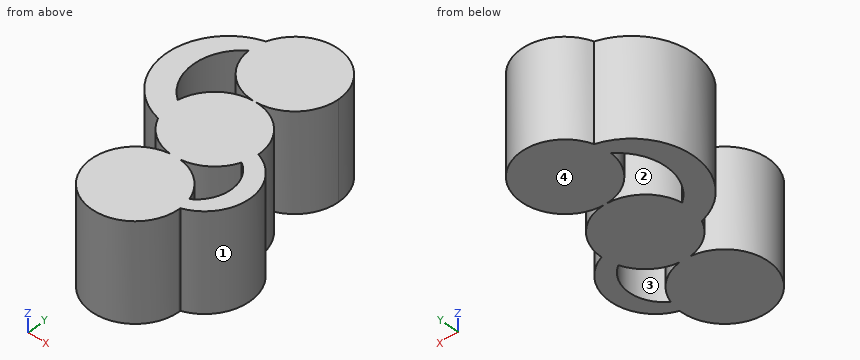
from build123d import *

# Parameters (mm, degrees)
F1_DEPTH = 25


with BuildPart() as f1:
    # F0 (on Top) → F1 (new body)
    with BuildSketch(Plane.XY):
        with BuildLine():
            ThreePointArc((-0.3111750606, 11.1956764013), (-7.4017548814, 8.4055948436), (-11.0663750249, 1.7249184932))
            ThreePointArc((-11.0663750249, 1.7249184932), (-11.0810170285, -1.6282080989), (-10.1024246207, -4.8353921022))
            ThreePointArc((-10.1024246207, -4.8353921022), (-6.5247892852, -9.1031381833), (-1.3339990852, -11.120271869))
            ThreePointArc((-1.3339990852, -11.120271869), (0, -11.040543738), (1.3339990852, -11.120271869))
            ThreePointArc((1.3339990852, -11.120271869), (6.9190712637, -8.8071818902), (10.4884666015, -3.9283671354))
            ThreePointArc((10.4884666015, -3.9283671354), (11.0206811481, -1.9961430389), (11.2, 0))
            ThreePointArc((11.2, 0), (8.0288592178, 7.808803984), (0.3111750606, 11.1956764013))
            ThreePointArc((0.3111750606, 11.1956764013), (0, 11.1913528025), (-0.3111750606, 11.1956764013))
        make_face()
        with BuildLine():
            ThreePointArc((-10.1024246207, -4.8353921022), (-11.0810170285, -1.6282080989), (-11.0663750249, 1.7249184932))
            ThreePointArc((-11.0663750249, 1.7249184932), (-16.1436885781, 11.6980871603), (-11.1803662832, 21.7284728944))
            ThreePointArc((-11.1803662832, 21.7284728944), (-11.10579848, 23.8409182968), (-10.6356586789, 25.9017323357))
            ThreePointArc((-10.6356586789, 25.9017323357), (-22.131772625, 10.3291078016), (-10.1024246207, -4.8353921022))
        make_face()
        with BuildLine():
            ThreePointArc((-11.1803662832, 21.7284728944), (-7.7941536491, 14.3482707506), (-0.3111750606, 11.1956764013))
            ThreePointArc((-0.3111750606, 11.1956764013), (0, 11.2), (0.3111750606, 11.1956764013))
            ThreePointArc((0.3111750606, 11.1956764013), (8.0288592178, 14.5825488185), (11.2, 22.3913528025))
            ThreePointArc((11.2, 22.3913528025), (1.777726469, 33.4493674797), (-10.6356586789, 25.9017323357))
            ThreePointArc((-10.6356586789, 25.9017323357), (-11.10579848, 23.8409182968), (-11.1803662832, 21.7284728944))
        make_face()
        with BuildLine():
            ThreePointArc((0.3111750606, 11.1956764013), (0, 11.2), (-0.3111750606, 11.1956764013))
            ThreePointArc((-0.3111750606, 11.1956764013), (0, 11.1913528025), (0.3111750606, 11.1956764013))
        make_face()
        with BuildLine():
            ThreePointArc((1.3339990852, -11.120271869), (0, -11.040543738), (-1.3339990852, -11.120271869))
            ThreePointArc((-1.3339990852, -11.120271869), (0, -11.2), (1.3339990852, -11.120271869))
        make_face()
        with BuildLine():
            ThreePointArc((1.3339990852, -11.120271869), (0, -11.2), (-1.3339990852, -11.120271869))
            ThreePointArc((-1.3339990852, -11.120271869), (-7.4330078113, -30.6185145471), (11.2, -22.240543738))
            ThreePointArc((11.2, -22.240543738), (11.1983095854, -22.0459610337), (11.193238852, -21.851437066))
            ThreePointArc((11.193238852, -21.851437066), (11.0205922894, -20.2439101733), (10.6182959163, -18.6779896214))
            ThreePointArc((10.6182959163, -18.6779896214), (7.0706515511, -13.5545845715), (1.3339990852, -11.120271869))
        make_face()
        with BuildLine():
            ThreePointArc((11.193238852, -21.851437066), (18.9710900132, -10.9281240657), (11.2, 0))
            ThreePointArc((11.2, 0), (11.0206811481, -1.9961430389), (10.4884666015, -3.9283671354))
            ThreePointArc((10.4884666015, -3.9283671354), (14.5159030008, -11.2682994191), (10.6182959163, -18.6779896214))
            ThreePointArc((10.6182959163, -18.6779896214), (11.0205922894, -20.2439101733), (11.193238852, -21.851437066))
        make_face()
    extrude(amount=F1_DEPTH)


solid = f1.part
CAD build for the part. Positions are in the model's coordinates, mm. Face numbers are marked on the shaded views. Round coordinates to 2 decimals unless told otherwise and drop trailing zeros. Write each loop counter-clockwise with the first axis right and the second up, starting at its lowest first coordinate (ties: lowest second). Pieces come first, ordered by that corner, then holes. Notation, with made-up numbers: (85, 18) -> (107, 18) arc R33 ccw to (107, 46) -> close; hole circle Ø8 at (87.5, 11.5). An arc over 180 degrees is marked (long way). Answer as a JSON object with one key per item and string values.
(1) Two-plate mould, pull along X, no slides. Class the marked faces 1, 2, 3 and 4: +X half, -X half, draft (parallel to the pull), parting line (faces both ways), or undercut.
Reported:
{"face 1": "+X half", "face 2": "undercut", "face 3": "undercut", "face 4": "draft"}
(2) Probe probe 1 along Y at (x, z) = (-5, 19.5); probe 2 along Y at (x, z) = (2, 19); probe 3 along X at (y, z) = (19, 5.75). List the from-to ranges inside material, lowest first. Write a range as [from, to].
Reported:
{"probe 1": "y = [-32.26, -12.22], [-10.02, 10.02], [12.37, 32.41]", "probe 2": "y = [-33.26, -11.22], [-11.02, 11.02], [11.37, 33.41]", "probe 3": "x = [-19.74, -13.83], [-10.67, 10.67]"}
(3) Band-saw the part on C-C, the plane y = 13. List the corners of the cut face in (x, z), then the cut area to 3 significant figures.
Reported:
{"outline": "(-21.95, 0) -> (-16.08, 0) -> (-16.08, 25) -> (-21.95, 25) -> close; (-6.1, 0) -> (6.1, 0) -> (6.1, 25) -> (-6.1, 25) -> close", "area": "452 mm^2"}
(4) Band-saw the part on B-B, the plane x = -8.5. List the corners of the cut face in (y, z).
Reported:
{"outline": "(-29.53, 0) -> (-14.95, 0) -> (-14.95, 25) -> (-29.53, 25) -> close; (-7.29, 0) -> (7.29, 0) -> (7.29, 25) -> (-7.29, 25) -> close; (15.1, 0) -> (29.68, 0) -> (29.68, 25) -> (15.1, 25) -> close"}
(5) Band-saw the part on D-D, the plane x = -3. List the corners of the cut face in (y, z), then the cut area to 3 significant figures.
Reported:
{"outline": "(-33.03, 0) -> (-11.45, 0) -> (-11.45, 25) -> (-33.03, 25) -> close; (-10.79, 0) -> (10.79, 0) -> (10.79, 25) -> (-10.79, 25) -> close; (11.6, 0) -> (33.18, 0) -> (33.18, 25) -> (11.6, 25) -> close", "area": "1,620 mm^2"}
(6) Band-saw the part on A-A, the plane z = 13.75. List the corners of the cut face in (x, y), then the cut area to 3 significant figures.
Reported:
{"outline": "(-10.64, 25.9) arc R15.92 ccw to (-10.1, -4.84) arc R11.2 ccw to (-1.33, -11.12) arc R11.2 ccw (long way) to (11.19, -21.85) arc R11.56 ccw to (11.2, 0) arc R11.2 ccw to (0.31, 11.2) arc R11.2 ccw (long way) to start; hole (-11.18, 21.73) arc R12.47 ccw to (-11.07, 1.72) arc R11.2 cw to (-0.31, 11.2) arc R11.2 cw to start; hole (1.33, -11.12) arc R11.2 cw to (10.62, -18.68) arc R8.84 ccw to (10.49, -3.93) arc R11.2 cw to start", "area": "1,450 mm^2"}
(7) Pin check, flat tips, straight feed: P1, Ø2, axis at x = -6, z = 4.5, coming from the -Y side; P2, Ø5, axis at y = 3, z = 6, coming from the +X side; P3, Ø4, axis at x = -12.5, y = 11.5, coming from the +Z side; P4, Ø2, axis at y = 12, z = 4.5, coming from the +X side. Stop position of each tip, or through.
Reported:
{"P1": "stops at y = -32.26", "P2": "stops at x = 11.19", "P3": "passes through", "P4": "stops at x = 6.1"}
